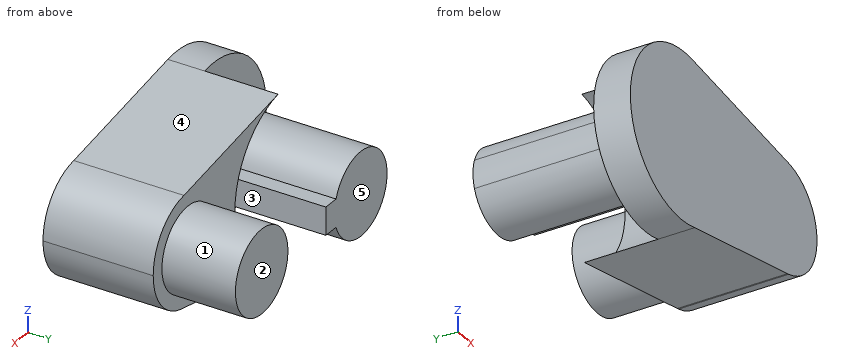
from build123d import *

# Parameters (mm, degrees)
F1_DEPTH = 63.5
F2_DEPTH = 12.7
F0_R     = 14.2875
F3_DEPTH = 38.1
F4_DEPTH = 63.5


with BuildPart() as f1:
    # F0 (on Front) → F1 (new body)
    with BuildSketch(Plane.XZ):
        with BuildLine():
            Line((-28.9843866844, 4.7399969062), (-2.0436183212, 4.7399969062))
            ThreePointArc((-2.0436183212, 4.7399969062), (-15.5140025028, 14.2649969062), (-28.9843866844, 4.7399969062))
        make_face()
        with BuildLine():
            ThreePointArc((-2.0436183212, -4.7850030938), (-1.4322630818, -2.4385476149), (-1.2265025028, -0.0225030938))
            ThreePointArc((-1.2265025028, -0.0225030938), (-1.4322630818, 2.3935414272), (-2.0436183212, 4.7399969062))
            Line((-2.0436183212, 4.7399969062), (-28.9843866844, 4.7399969062))
            ThreePointArc((-28.9843866844, 4.7399969062), (-29.8015025028, -0.0225030938), (-28.9843866844, -4.7850030938))
            Line((-28.9843866844, -4.7850030938), (-2.0436183212, -4.7850030938))
        make_face()
        with BuildLine():
            ThreePointArc((-28.9843866844, -4.7850030938), (-15.5140025028, -14.3100030938), (-2.0436183212, -4.7850030938))
            Line((-2.0436183212, -4.7850030938), (-28.9843866844, -4.7850030938))
        make_face()
        with BuildLine():
            ThreePointArc((-2.0436183212, 4.7399969062), (-1.4322630818, 2.3935414272), (-1.2265025028, -0.0225030938))
            ThreePointArc((-1.2265025028, -0.0225030938), (-1.4322630818, -2.4385476149), (-2.0436183212, -4.7850030938))
            Line((-2.0436183212, -4.7850030938), (3.5359974972, -4.7850030938))
            Line((3.5359974972, -4.7850030938), (3.5359974972, 4.7399969062))
            Line((3.5359974972, 4.7399969062), (-2.0436183212, 4.7399969062))
        make_face()
    extrude(amount=-F1_DEPTH)

    # F0 (on Front) → F2 (join)
    with BuildSketch(Plane.XZ):
        with BuildLine():
            ThreePointArc((-9.1005831185, -27.8684844341), (6.8443749417, -17.8167039201), (13.0609974972, -0.0225030938))
            ThreePointArc((13.0609974972, -0.0225030938), (6.4072485943, 18.3075098722), (-10.4553192367, 28.1011586274))
            ThreePointArc((-10.4553192367, 28.1011586274), (-44.0806355021, -0.713953805), (-9.1005831185, -27.8684844341))
        make_face()
        with BuildLine():
            ThreePointArc((-28.9843866844, 4.7399969062), (-15.5140025028, 14.2649969062), (-2.0436183212, 4.7399969062))
            Line((-2.0436183212, 4.7399969062), (3.5359974972, 4.7399969062))
            Line((3.5359974972, 4.7399969062), (3.5359974972, -4.7850030938))
            Line((3.5359974972, -4.7850030938), (-2.0436183212, -4.7850030938))
            ThreePointArc((-2.0436183212, -4.7850030938), (-15.5140025028, -14.3100030938), (-28.9843866844, -4.7850030938))
            Line((-28.9843866844, -4.7850030938), (-34.5640025028, -4.7850030938))
            Line((-34.5640025028, -4.7850030938), (-34.5640025028, 4.7399969062))
            Line((-34.5640025028, 4.7399969062), (-28.9843866844, 4.7399969062))
        make_face(mode=Mode.SUBTRACT)
        with BuildLine():
            ThreePointArc((-28.9843866844, -4.7850030938), (-29.8015025028, -0.0225030938), (-28.9843866844, 4.7399969062))
            Line((-28.9843866844, 4.7399969062), (-34.5640025028, 4.7399969062))
            Line((-34.5640025028, 4.7399969062), (-34.5640025028, -4.7850030938))
            Line((-34.5640025028, -4.7850030938), (-28.9843866844, -4.7850030938))
        make_face()
    extrude(amount=-F2_DEPTH)

    # F0 (on Front) → F3 (join)
    with BuildSketch(Plane.XZ):
        with BuildLine():
            ThreePointArc((-10.4553192367, 28.1011586274), (6.4072485943, 18.3075098722), (13.0609974972, -0.0225030938))
            ThreePointArc((13.0609974972, -0.0225030938), (6.8443749417, -17.8167039201), (-9.1005831185, -27.8684844341))
            Line((-9.1005831185, -27.8684844341), (41.4850136025, -18.8309540294))
            ThreePointArc((41.4850136025, -18.8309540294), (19.4144080306, -0.3829607102), (40.7712014453, 18.8868982113))
            Line((40.7712014453, 18.8868982113), (-10.4553192367, 28.1011586274))
        make_face()
        with BuildLine():
            ThreePointArc((57.5109974972, -0.0225030938), (52.7247958204, 12.6047118562), (40.7712014453, 18.8868982113))
            ThreePointArc((40.7712014453, 18.8868982113), (19.4144080306, -0.3829607102), (41.4850136025, -18.8309540294))
            Line((41.4850136025, -18.8309540294), (42.136745961, -18.7145167154))
            ThreePointArc((42.136745961, -18.7145167154), (53.1736707457, -12.1237322001), (57.5109974972, -0.0225030938))
        make_face()
        with Locations((38.4609974972, -0.0225030938)):
            Circle(F0_R, mode=Mode.SUBTRACT)
    extrude(amount=-F3_DEPTH)

    # F0 (on Front) → F4 (join)
    with BuildSketch(Plane.XZ):
        with Locations((38.4609974972, -0.0225030938)):
            Circle(F0_R)
    extrude(amount=-F4_DEPTH)


solid = f1.part
Here's how the part is built. I have some questions about the finished solid (model axes, mm). Face numbers are marked on the shaded views. A direction names the side the tool comes from. Round coordinates to 2 decimals unless told otherwise and drop trailing zeros. Order: outer loops, then holes, each group sorted by start corner. A loop starts at its lowest first (then second) coordinate and runs counter-clockwise, first axis right, second up. Notation, with made-up numbers: (52.25, -30.75) -> (80.25, -30.75) arc R13 cw to (80.25, -21.75) -> close; hole circle Ø6 at (-23, -20.75). An arc over 180 degrees is marked (long way). Use CSV: the item, a comma, the result in double quotes.
1. I want a section at C-C on z = -13. List the corners of the cut face in (x, y) for me, and give its area (3 significant figures).
Recorded:
outline,"(-40.97, 0) -> (52.41, 0) -> (52.41, 38.1) -> (44.44, 38.1) -> (44.44, 63.5) -> (32.48, 63.5) -> (32.48, 38.1) -> (9.94, 38.1) -> (9.94, 12.7) -> (-9.54, 12.7) -> (-9.54, 63.5) -> (-21.49, 63.5) -> (-21.49, 12.7) -> (-40.97, 12.7) -> close"
area,"3,180 mm2"
2. I need wall thicknesses on line 1 along Z through (x, y) = (2, 35) (3 decimals); line 2 along Y through (x, z) = (0.5, -24.5); line 3 along Z through (x, y) = (-1.5, 26) (3 decimals). Which ranges of each line are inside material? Lowest first, please.
Recorded:
line 1,"z = -25.885 to -22.601, -4.785 to 4.74, 22.556 to 25.861"
line 2,"y = 0 to 38.1"
line 3,"z = -26.511 to -24.925, -4.785 to 4.74, 24.88 to 26.49"
3. Which directions (+Z, -Z, +X, -X, +Y, -Y) give clear straight access to the entire face, cutting with the end or side of a thin tool? Please do the marked faces 1 and 2.
Recorded:
face 1,"+Y"
face 2,"+Z, -Z, +X, -X, +Y"
4. I'm going to push flat-ended pins straight in: P1, Ø6, axis at x = 43.5, z = 13, coming from the -Y side; P2, Ø3, axis at y = 48.5, z = -6, coming from the +X side; P3, Ø8, axis at x = -17.5, z = 20, coming from the +Y side; P4, Ø7.5, axis at y = 41, z = -2.5, coming from the +X side. Where does each tip first touch, or does it pass through?
Recorded:
P1,"stops at y = 0"
P2,"stops at x = 52.03"
P3,"stops at y = 12.7"
P4,"stops at x = 57.51"
5. I want a section at B-B on x = 5.5. List the corners of the cut face in (y, z) for me.
Recorded:
outline,"(0, -25.26) -> (38.1, -25.26) -> (38.1, -19.39) -> (12.7, -19.39) -> (12.7, 19.34) -> (38.1, 19.34) -> (38.1, 25.23) -> (0, 25.23) -> close"
6. Thinking about a two-plate mould opening in X: for the marked faces 3, 4 and 5, which applies, pulls with the +X half, pulls with the -X half, needs draft (parallel to the pull), parting line crosses it, or undercut?
Recorded:
face 3,"undercut"
face 4,"pulls with the +X half"
face 5,"needs draft"
7. I want a section at A-A on y = 49.5. List the corners of the cut face in (x, z) for me (1 decimal).
Recorded:
outline,"(-2, -4.8) -> (3.5, -4.8) -> (3.5, 4.7) -> (-2, 4.7) arc R14.3 ccw (long way) to start; circle Ø28.6 at (38.5, 0)"
